```python
from build123d import *

# Parameters (mm, degrees)
F0_R     = 5.25
F1_DEPTH = 6
F0_R_2   = 60.5
F2_DEPTH = 3
F3_SIZE  = 1.5


with BuildPart() as f1:
    # F0 (on Top) → F1 (new body)
    with BuildSketch(Plane.XY):
        with BuildLine():
            ThreePointArc((7.5, 49.4342998332), (37.9143772203, 32.596012026), (50, 0))
            ThreePointArc((50, 0), (49.1328198544, -9.2717858665), (46.5613594739, -18.2219593882))
            Line((46.5613594739, -18.2219593882), (53.7760869447, -22.3873842357))
            ThreePointArc((53.7760869447, -22.3873842357), (57.1205723209, -11.4150215828), (58.25, 0))
            ThreePointArc((58.25, 0), (43.7603559172, 38.4459848359), (7.5, 57.7651495281))
            Line((7.5, 57.7651495281), (7.5, 49.4342998332))
        make_face()
        with BuildLine():
            ThreePointArc((0, 50), (3.7606520937, 49.8583743801), (7.5, 49.4342998332))
            Line((7.5, 49.4342998332), (7.5, 57.7651495281))
            Line((7.5, 57.7651495281), (-7.5, 57.7651495281))
            Line((-7.5, 57.7651495281), (-7.5, 49.4342998332))
            ThreePointArc((-7.5, 49.4342998332), (-3.7606520937, 49.8583743801), (0, 50))
        make_face()
        with BuildLine():
            ThreePointArc((-46.5613594739, -18.2219593882), (-43.3012701892, 25), (-7.5, 49.4342998332))
            Line((-7.5, 49.4342998332), (-7.5, 57.7651495281))
            ThreePointArc((-7.5, 57.7651495281), (-50.4459797704, 29.125), (-53.7760869447, -22.3873842357))
            Line((-53.7760869447, -22.3873842357), (-46.5613594739, -18.2219593882))
        make_face()
        with BuildLine():
            Line((-46.2760869447, -35.3777652924), (-39.0613594739, -31.212340445))
            ThreePointArc((-39.0613594739, -31.212340445), (-43.3012701892, -25), (-46.5613594739, -18.2219593882))
            Line((-46.5613594739, -18.2219593882), (-53.7760869447, -22.3873842357))
            ThreePointArc((-53.7760869447, -22.3873842357), (-50.4459797704, -29.125), (-46.2760869447, -35.3777652924))
        make_face()
        with BuildLine():
            Line((46.2760869447, -35.3777652924), (39.0613594739, -31.212340445))
            ThreePointArc((39.0613594739, -31.212340445), (0, -50), (-39.0613594739, -31.212340445))
            Line((-39.0613594739, -31.212340445), (-46.2760869447, -35.3777652924))
            ThreePointArc((-46.2760869447, -35.3777652924), (0, -58.25), (46.2760869447, -35.3777652924))
        make_face()
        with BuildLine():
            Line((53.7760869447, -22.3873842357), (46.5613594739, -18.2219593882))
            ThreePointArc((46.5613594739, -18.2219593882), (43.3012701892, -25), (39.0613594739, -31.212340445))
            Line((39.0613594739, -31.212340445), (46.2760869447, -35.3777652924))
            ThreePointArc((46.2760869447, -35.3777652924), (50.4459797704, -29.125), (53.7760869447, -22.3873842357))
        make_face()
        with BuildLine():
            Line((-7.5, 57.7651495281), (7.5, 57.7651495281))
            ThreePointArc((7.5, 57.7651495281), (0, 58.25), (-7.5, 57.7651495281))
        make_face()
        with BuildLine():
            Line((7.5, 40), (7.5, 49.4342998332))
            ThreePointArc((7.5, 49.4342998332), (3.7606520937, 49.8583743801), (0, 50))
            Line((0, 50), (0, 47.5))
            ThreePointArc((0, 47.5), (5.3033008589, 45.3033008589), (7.5, 40))
        make_face()
        with BuildLine():
            Line((0, 47.5), (0, 50))
            ThreePointArc((0, 50), (-3.7606520937, 49.8583743801), (-7.5, 49.4342998332))
            Line((-7.5, 49.4342998332), (-7.5, 40))
            ThreePointArc((-7.5, 40), (-5.3033008589, 45.3033008589), (0, 47.5))
        make_face()
        with BuildLine():
            ThreePointArc((-7.5, 40), (0, 32.5), (7.5, 40))
            ThreePointArc((7.5, 40), (5.3033008589, 45.3033008589), (0, 47.5))
            ThreePointArc((0, 47.5), (-5.3033008589, 45.3033008589), (-7.5, 40))
        make_face()
        with BuildLine():
            ThreePointArc((5.25, 40), (-3.7123106012, 36.2876893988), (0, 45.25))
            ThreePointArc((0, 45.25), (3.7123106012, 43.7123106012), (5.25, 40))
        make_face(mode=Mode.SUBTRACT)
        with BuildLine():
            ThreePointArc((39.0613594739, -31.212340445), (43.3012701892, -25), (46.5613594739, -18.2219593882))
            Line((46.5613594739, -18.2219593882), (38.3910161948, -13.5048094967))
            ThreePointArc((38.3910161948, -13.5048094967), (41.1362066923, -16.2500000217), (42.1410161514, -20))
            ThreePointArc((42.1410161514, -20), (38.3910161049, -26.4951905552), (30.8910160584, -26.4951904747))
            Line((30.8910160584, -26.4951904747), (39.0613594739, -31.212340445))
        make_face()
        with BuildLine():
            ThreePointArc((42.1410161514, -20), (41.1362066923, -16.2500000217), (38.3910161948, -13.5048094967))
            ThreePointArc((38.3910161948, -13.5048094967), (28.1458256624, -16.2499999318), (30.8910160584, -26.4951904747))
            ThreePointArc((30.8910160584, -26.4951904747), (38.3910161049, -26.4951905552), (42.1410161514, -20))
        make_face()
        with Locations((34.6410161514, -20)):
            Circle(F0_R, mode=Mode.SUBTRACT)
        with BuildLine():
            ThreePointArc((-38.3910159202, -13.5048093381), (-41.1362067455, -23.7499998861), (-30.891016148, -26.4951905264))
            ThreePointArc((-30.891016148, -26.4951905264), (-28.145825622, -23.7499999983), (-27.1410161514, -20))
            ThreePointArc((-27.1410161514, -20), (-30.8910160358, -13.5048095384), (-38.3910159202, -13.5048093381))
        make_face()
        with Locations((-34.6410161514, -20)):
            Circle(F0_R, mode=Mode.SUBTRACT)
        with BuildLine():
            ThreePointArc((-46.5613594739, -18.2219593882), (-43.3012701892, -25), (-39.0613594739, -31.212340445))
            Line((-39.0613594739, -31.212340445), (-30.891016148, -26.4951905264))
            ThreePointArc((-30.891016148, -26.4951905264), (-41.1362067455, -23.7499998861), (-38.3910159202, -13.5048093381))
            Line((-38.3910159202, -13.5048093381), (-46.5613594739, -18.2219593882))
        make_face()
        with BuildLine():
            Line((7.5, 22.2348504719), (7.5, 40))
            ThreePointArc((7.5, 40), (0, 32.5), (-7.5, 40))
            Line((-7.5, 40), (-7.5, 22.2348504719))
            Line((-7.5, 22.2348504719), (7.5, 22.2348504719))
        make_face()
        with BuildLine():
            ThreePointArc((30.8910160584, -26.4951904747), (28.1458256624, -16.2499999318), (38.3910161948, -13.5048094967))
            Line((38.3910161948, -13.5048094967), (23.005945358, -4.6222347076))
            Line((23.005945358, -4.6222347076), (7.5, 22.2348504719))
            Line((7.5, 22.2348504719), (-7.5, 22.2348504719))
            Line((-7.5, 22.2348504719), (-23.005945358, -4.6222347076))
            Line((-23.005945358, -4.6222347076), (-38.3910159202, -13.5048093381))
            ThreePointArc((-38.3910159202, -13.5048093381), (-30.8910160358, -13.5048095384), (-27.1410161514, -20))
            ThreePointArc((-27.1410161514, -20), (-28.145825622, -23.7499999983), (-30.891016148, -26.4951905264))
            Line((-30.891016148, -26.4951905264), (-15.505945358, -17.6126157643))
            Line((-15.505945358, -17.6126157643), (15.505945358, -17.6126157643))
            Line((15.505945358, -17.6126157643), (30.8910160584, -26.4951904747))
        make_face()
        with BuildLine():
            ThreePointArc((0, 10), (7.0710678119, 7.0710678119), (10, 0))
            ThreePointArc((10, 0), (7.0710678119, -7.0710678119), (0, -10))
            ThreePointArc((0, -10), (-7.0710678119, -7.0710678119), (-10, 0))
            ThreePointArc((-10, 0), (-7.0710678119, 7.0710678119), (0, 10))
        make_face(mode=Mode.SUBTRACT)
    extrude(amount=F1_DEPTH)

    # F0 (on Top) → F2 (join)
    with BuildSketch(Plane.XY):
        Circle(F0_R_2)
        with BuildLine():
            ThreePointArc((-7.5, 57.7651495281), (0, 58.25), (7.5, 57.7651495281))
            ThreePointArc((7.5, 57.7651495281), (43.7603559172, 38.4459848359), (58.25, 0))
            ThreePointArc((58.25, 0), (57.1205723209, -11.4150215828), (53.7760869447, -22.3873842357))
            ThreePointArc((53.7760869447, -22.3873842357), (50.4459797704, -29.125), (46.2760869447, -35.3777652924))
            ThreePointArc((46.2760869447, -35.3777652924), (0, -58.25), (-46.2760869447, -35.3777652924))
            ThreePointArc((-46.2760869447, -35.3777652924), (-50.4459797704, -29.125), (-53.7760869447, -22.3873842357))
            ThreePointArc((-53.7760869447, -22.3873842357), (-50.4459797704, 29.125), (-7.5, 57.7651495281))
        make_face(mode=Mode.SUBTRACT)
        with BuildLine():
            ThreePointArc((-7.5, 0), (-5.3033008589, 5.3033008589), (0, 7.5))
            Line((0, 7.5), (0, 10))
            ThreePointArc((0, 10), (-7.0710678119, 7.0710678119), (-10, 0))
            Line((-10, 0), (-7.5, 0))
        make_face()
        with BuildLine():
            Line((10, 0), (7.5, 0))
            ThreePointArc((7.5, 0), (5.3033008589, -5.3033008589), (0, -7.5))
            Line((0, -7.5), (0, -10))
            ThreePointArc((0, -10), (7.0710678119, -7.0710678119), (10, 0))
        make_face()
    extrude(amount=F2_DEPTH)

    # F3
    f3_edges = [f1.edges().sort_by_distance(p)[0] for p in [
        (-7.5, -57.76515, 6),
    ]]
    chamfer(f3_edges, length=F3_SIZE)


solid = f1.part
```
Geometry: final body of the model. Coordinates: model frame, mm. A direction names the side the tool comes from. Give positions to 0.01 mm unless a question says otherwise; leave off trailing zeros. Loops run counter-clockwise (first coordinate to the right, second up) from the corner with the lowest first, then second, coordinate; pieces in that order, holes last. Notation, with made-up numbers: (67.5, 18.25) -> (113.5, 18.25) arc R27 cw to (113.5, 39.25) -> close; hole circle Ø11 at (14, -1). An arc over 180 degrees is marked (long way). Use one line per item in the form item = value.
Item 1: Section query B-B on y = 47. Give the number of separate pieces and of enclosed holes in the cut face, and give its area (3 significant figures).
A:
separate_pieces = 3
enclosed_holes = 0
area = 316 mm^2
Item 2: Line query: probe 1 along X at (y, z) = (40, 2); probe 2 along X at (y, z) = (31.5, 3.5); probe 3 along Y at (x, z) = (-20, 1.7). Output: solid intervals per line, ascending.
A:
probe_1 = -45.39 to -30, -7.5 to -5.25, 5.25 to 7.5, 30 to 45.39
probe_2 = -49 to -38.83, -7.5 to 7.5, 38.83 to 49
probe_3 = -57.1 to -45.83, -20.21 to 0.58, 45.83 to 57.1
Item 3: Section query A-A on z = 1.45. Output: boundary loops of the cut face in (x, y), and give its area (3 significant figures).
A:
outline = circle Ø121 at (0, 0); hole (-46.56, -18.22) -> (-23.01, -4.62) -> (-7.5, 22.23) -> (-7.5, 49.43) arc R50 ccw to start; hole circle Ø10.5 at (-34.64, -20); hole (-39.06, -31.21) arc R50 ccw to (39.06, -31.21) -> (15.51, -17.61) -> (-15.51, -17.61) -> close; hole (-10, 0) arc R10 ccw to (0, -10) -> (0, -7.5) arc R7.5 ccw to (7.5, 0) -> (10, 0) arc R10 ccw to (0, 10) -> (0, 7.5) arc R7.5 ccw to (-7.5, 0) -> close; hole circle Ø10.5 at (0, 40); hole (7.5, 22.23) -> (23.01, -4.62) -> (46.56, -18.22) arc R50 ccw to (7.5, 49.43) -> close; hole circle Ø10.5 at (34.64, -20)
area = 5,700 mm^2
Item 4: Access query for faces 1 (the face through (6, -5, 3)), 2 (the face through (7.5, 36, 3)), 3 (the face through (8, -8, 6)). Directions: +Z, -Z, +X, -X, +Y, -Y. A direction counts if a zero-diameter tool reaches every point of the face in a straight line with its end or side. Return the directions, or none.
A:
face_1 = +Z
face_2 = +Z, -Z
face_3 = +Z, +X, -X, +Y, -Y
Item 5: Pin query (flat end, axial travel): P1, Ø3, axis at y = 34.5, z = 3.5, coming from the -X side; P2, Ø6.5, axis at x = 34.64, y = -20, coming from the +Z side; P3, Ø1, axis at y = 45.5, z = 4, coming from the -X side; P4, Ø0.8, axis at x = 9, z = 1.5, coming from the +Y side. Return the tip coordinate at first contact, or that it passes through.
A:
P1 = -50.65
P2 = through
P3 = -36.99
P4 = 59.89
Item 6: Draft query along X for faces 4 (the face through (-29.633, -18.423, 2.958)), 5 (the face through (-32, 50, 3)), 6 (the face through (-13.12, -59.06, 1.48)). Return one class per face: pulls with the +X half, pulls with the -X half, needs draft (parallel to the pull), parting line crosses it, or undercut.
A:
face_4 = undercut
face_5 = needs draft
face_6 = parting line crosses it
